Can you work these out from the drawing? Everything is in mm from the part's minimum corner. A direction names the side the tool comes from. Round coordinates to 2 decimals unless told otherwise and drop trailing zeros. Write each loop counter-clockwise with the first axis right and the second up, starting at its lowest first coordinate (ties: lowest second). Pieces come first, ordered by that corner, then holes. Notation, with made-up numbers: (48.25, 62) -> (60.25, 62) arc R23 cw to (60.25, 85) -> close; hole circle Ø7 at (26.25, -28.75). An arc over 180 degrees is marked (long way). Answer as CSV lines item,"result". Start each with the question number.
Q1. If we mould it in two halves opening along X, with no side actions, what happens to the marked faces 4, 5 and 6? For each: pulls with the +X half, pulls with the -X half, needs draft (parallel to the pull), parting line crosses it, or undercut.
Q2. Imagine slicing it at A-A on z = 7.5. Please give me the cut outline in (x, y).
Q3. For the marked faces 1, 2 and 3, which set-ups out of +Z, -Z, +X, -X, +Y, -Y let a thin tool reach every point of the face, with its end or its side?
Q4. If I drill on line 1 (X direction, y = 6, z = 10); line 2 (X direction, y = 21, z = 4.25); line 3 (Z direction, x = 25, y = 8), over which ranges is the centre line in solid material (lowest first)? Write a range as [from, to].
Q5. Will these pins go through, and if not, where does the flat tip stop? pin 1 Ø2 at (y, z) = (16, 9.5) entering from +X; pin 2 Ø1 at (x, z) = (2, 6) entering from +Y; pin 3 Ø1.5 at (x, z) = (21.5, 9) entering from -Y.
Q6. Imagine slicing it at D-D on x = 19. Please give me the cut outline in (y, z).
Q7. Imagine slicing it at B-B on x = 6. Please give me the cut outline in (y, z).
Q8. Imagine slicing it at C-C on y = 33. Please give me the cut outline in (x, z).
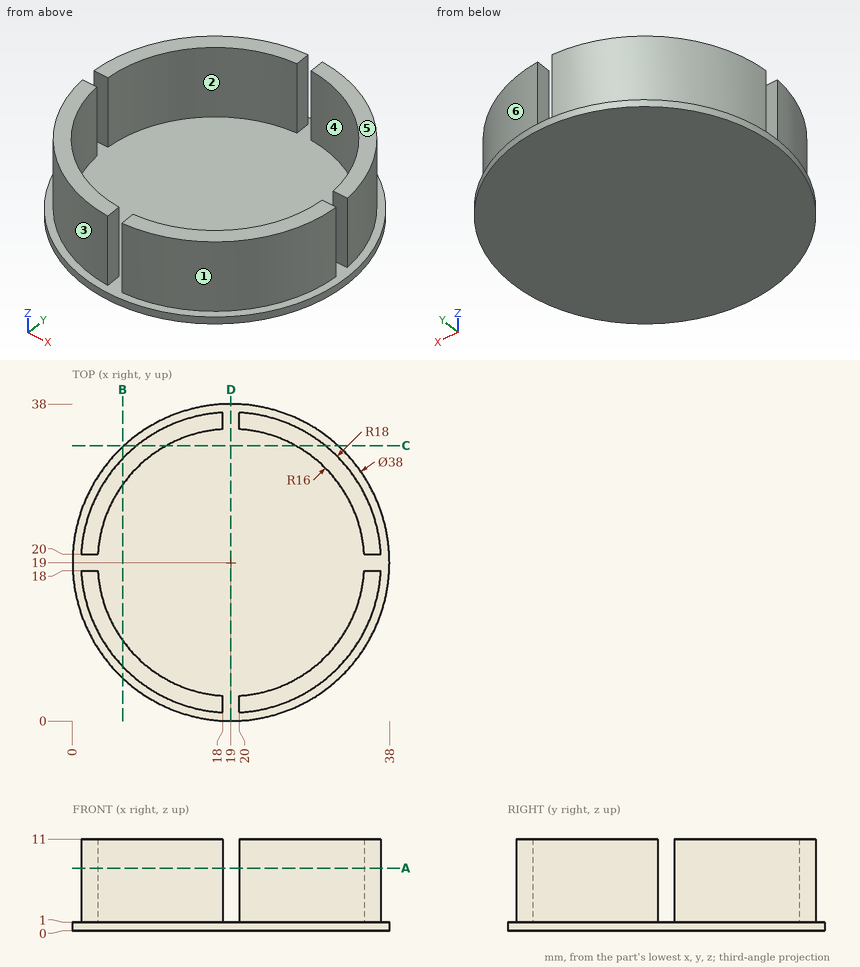
Checks:
1,face 4,"undercut"
1,face 5,"needs draft"
1,face 6,"pulls with the +X half"
2,outline,"(1.03, 18) arc R18 ccw to (18, 1.03) -> (18, 3.03) arc R16 cw to (3.03, 18) -> close; (1.03, 20) -> (3.03, 20) arc R16 cw to (18, 34.97) -> (18, 36.97) arc R18 ccw to start; (20, 1.03) arc R18 ccw to (36.97, 18) -> (34.97, 18) arc R16 cw to (20, 3.03) -> close; (20, 34.97) arc R16 cw to (34.97, 20) -> (36.97, 20) arc R18 ccw to (20, 36.97) -> close"
3,face 1,"+Z, +X, -Y"
3,face 2,"+Z"
3,face 3,"+Z, -X, -Y"
4,line 1,"[6.55, 9.67], [28.33, 31.45]"
4,line 2,"[1.11, 3.13], [34.87, 36.89]"
4,line 3,"[0, 1]"
5,pin 1,"x = 36.89"
5,pin 2,"y = 26.19"
5,pin 3,"y = 1.09"
6,outline,"(0, 0) -> (38, 0) -> (38, 1) -> (0, 1) -> close"
7,outline,"(5.14, 0) -> (32.86, 0) -> (32.86, 1) -> (31.45, 1) -> (31.45, 11) -> (28.33, 11) -> (28.33, 1) -> (9.67, 1) -> (9.67, 11) -> (6.55, 11) -> (6.55, 1) -> (5.14, 1) -> close"
8,outline,"(6.15, 0) -> (31.85, 0) -> (31.85, 1) -> (30.31, 1) -> (30.31, 11) -> (26.75, 11) -> (26.75, 1) -> (11.25, 1) -> (11.25, 11) -> (7.69, 11) -> (7.69, 1) -> (6.15, 1) -> close"
